```python
from build123d import *

# Parameters (mm, degrees)
PAD_DEPTH       = 8
SKETCH001_R     = 6.75
PAD001_DEPTH    = 7
SKETCH002_R     = 5.05
POCKET_DEPTH    = 15.001
SKETCH003_R     = 3.5
PAD002_DEPTH    = 5
PAD003_DEPTH    = 10
SKETCH005_W     = 15.5
SKETCH005_H     = 8
PAD004_DEPTH    = 9
SKETCH006_R     = 2.5
POCKET001_DEPTH = 31.001
POCKET002_DEPTH = 3.1


with BuildPart() as part:
    # Sketch → Pad (new body)
    with BuildSketch(Plane.XZ):
        with BuildLine():
            ThreePointArc((-28, 11), (-39, 0), (-28, -11))
            Line((-28, -11), (28, -11))
            ThreePointArc((28, -11), (39, 0), (28, 11))
            Line((-28, 11), (28, 11))
        make_face()
    extrude(amount=PAD_DEPTH)

    # Sketch001 (on Face5 of Pad) → Pad001 (join)
    with BuildSketch(Plane(origin=(0, 0, 0), x_dir=(1, 0, 0), z_dir=(0, 1, 0))):
        with Locations((-28, 0)):
            Circle(SKETCH001_R)
        with Locations((28, 0)):
            Circle(SKETCH001_R)
    extrude(amount=PAD001_DEPTH)

    # Sketch002 (on Face5 of Pad001) → Pocket (cut, through all)
    with BuildSketch(Plane.XZ.offset(8)):
        with Locations((-28, 0)):
            Circle(SKETCH002_R)
        with Locations((28, 0)):
            Circle(SKETCH002_R)
    extrude(amount=-POCKET_DEPTH, mode=Mode.SUBTRACT)

    # Sketch003 (on DatumPlane) → Pad002 (join)
    with BuildSketch(Plane.XY.offset(3.75)):
        with BuildLine():
            Line((-17.5, -8), (-6.180484, -29.286582))
            ThreePointArc((-6.180484, -29.286582), (0, -33), (6.180484, -29.286582))
            Line((17.5, -8), (6.180484, -29.286582))
            Line((-17.5, -8), (17.5, -8))
        make_face()
        with Locations((0, -26)):
            Circle(SKETCH003_R, mode=Mode.SUBTRACT)
    pad002 = extrude(amount=PAD002_DEPTH)

    # Mirrored: Pad002 across XY
    add(pad002.mirror(Plane.XY))

    # Sketch004 → Pad003 (join, symmetric)
    with BuildSketch(Plane.YZ):
        Polygon((0, 8), (0, -8), (20, 3), (20, 8), align=None)
    extrude(amount=PAD003_DEPTH, both=True)

    # Sketch005 (on Face2 of Pad003) → Pad004 (join)
    with BuildSketch(Plane(origin=(0, 0, 11), x_dir=(-1, 0, 0), z_dir=(0, 0, 1))):
        with Locations((0, 4)):
            Rectangle(SKETCH005_W, SKETCH005_H)
    extrude(amount=PAD004_DEPTH)

    # Sketch006 (on Face3 of Pad004) → Pocket001 (cut, through all)
    with BuildSketch(Plane(origin=(0, 0, -11), x_dir=(1, 0, 0), z_dir=(0, 0, -1))):
        with Locations((-4, 4)):
            Circle(SKETCH006_R)
        with Locations((4, 4)):
            Circle(SKETCH006_R)
    extrude(amount=-POCKET001_DEPTH, mode=Mode.SUBTRACT)

    # Sketch007 (on Face3 of Pocket001) → Pocket002 (cut)
    with BuildSketch(Plane(origin=(0, 0, -11), x_dir=(1, 0, 0), z_dir=(0, 0, -1))):
        Polygon((-0.55, 5.991858), (-4, 7.983717), (-7.45, 5.991858), (-7.45, 2.008142), (-4, 0.016283), (-0.55, 2.008142), align=None)
        Polygon((4, 7.983717), (0.55, 5.991858), (0.55, 2.008142), (4, 0.016283), (7.45, 2.008142), (7.45, 5.991858), align=None)
    extrude(amount=-POCKET002_DEPTH, mode=Mode.SUBTRACT)


solid = part.part
```
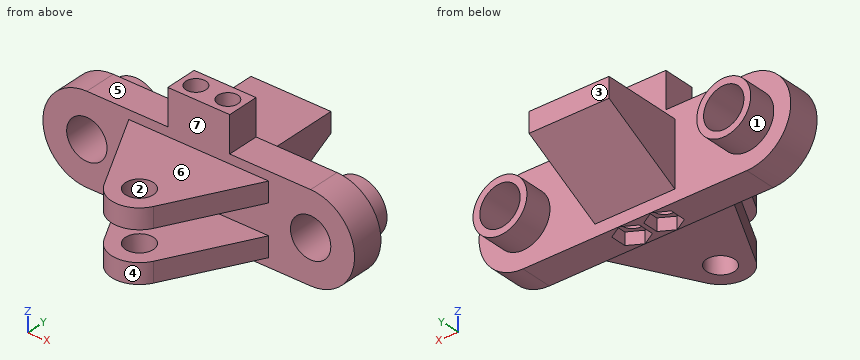
Could you check a few things on this model? Use its own coordinates, in mm. Face numbers are marked on the shaded views. A direction names the side the tool comes from. Round coordinates to 2 decimals unless told otherwise and drop trailing zeros. Loops run counter-clockwise (first coordinate to the right, second up) from the corner with the lowest first, then second, coordinate; pieces in that order, holes last.
Q1. Thinking about a two-plate mould opening in Y: for the marked faces 1, 2, 3 and 4, which applies, pulls with the +Y half, pulls with the -Y half, needs draft (parallel to the pull), parting line crosses it, or undercut?
Q2. Please list where these lines run through material, in increasing order: L1, parallel to Z at x = -4, y = -25.5; L2, parallel to Y at x = 0, z = 5.75; L3, parallel to Z at x = 28, y = 2.5.
Q3. On a 3-axis mill with a long thin cutter (end or side, diameter ignored), from which of +Z, -Z, +X, -X, +Y, -Y can I reach the whole of each face in a straight line? I mean the marked faces 5, 6 and 7. Say none if no direction works.
Q4. For P1, Ø6, axis at y = 13, z = 3, coming from the +X side; P2, Ø6, axis at y = 9, z = 0, coming from the +X side; P3, Ø0.9, axis at y = -4, z = -9.5, coming from the +X side; P4, Ø10, axis at x = 1.5, z = -3.5, coming from the -Y side, each with a flat end and sliding along its axis, tell me the tip position at first contact or that it passes through.
Q5. I want a section at D-D (y = -17). Write out the boundary of the cut face in (x, z), and give its area (3 significant figures).
Q6. I want a section at B-B (x = -24). Write out the boundary of the cut face in (y, z), and give its area (3 significant figures).
Q7. I want a section at C-C (z = 16). Write out the boundary of the cut face in (x, y), and give its area (3 significant figures).
Q8. I want a section at A-A (y = -4). Write out the boundary of the cut face in (x, z), and give its area (3 significant figures).
Answer below:
1. face 1: needs draft
1. face 2: undercut
1. face 3: pulls with the +Y half
1. face 4: pulls with the -Y half
2. L1: z = -8.75 to -3.75, 3.75 to 8.75
2. L2: y = -33 to -29.5, -22.5 to 20
2. L3: z = -6.75 to -5.05, 5.05 to 6.75
3. face 5: +Z, -X, +Y, -Y
3. face 6: +Z, +X, -X, -Y
3. face 7: -Y
4. P1: stops at x = 10
4. P2: stops at x = 34.75
4. P3: stops at x = 34.25
4. P4: stops at y = -33
5. outline: (-12.71, -8.75) - (12.71, -8.75) - (12.71, -3.75) - (-12.71, -3.75) - close; (-12.71, 3.75) - (12.71, 3.75) - (12.71, 8.75) - (-12.71, 8.75) - close
5. area: 254 mm2
6. outline: (-8, -11) - (0, -11) - (0, -5.44) - (7, -5.44) - (7, -3.08) - (-8, -3.08) - close; (-8, 3.08) - (7, 3.08) - (7, 5.44) - (0, 5.44) - (0, 11) - (-8, 11) - close
6. area: 160 mm2
7. outline: (-7.75, -8) - (7.75, -8) - (7.75, 0) - (-7.75, 0) - close; hole circle Ø5 at (-4, -4); hole circle Ø5 at (4, -4)
7. area: 84.7 mm2
8. outline: (-28, -11) - (-7.45, -11) - (-7.45, -7.9) - (-6.5, -7.9) - (-6.5, 20) - (-7.75, 20) - (-7.75, 11) - (-28, 11) arc R11 ccw to start; (-1.5, -7.9) - (-0.55, -7.9) - (-0.55, -11) - (0.55, -11) - (0.55, -7.9) - (1.5, -7.9) - (1.5, 20) - (-1.5, 20) - close; (6.5, -7.9) - (7.45, -7.9) - (7.45, -11) - (28, -11) arc R11 ccw to (28, 11) - (7.75, 11) - (7.75, 20) - (6.5, 20) - close; hole circle Ø10.1 at (-28, 0); hole circle Ø10.1 at (28, 0)
8. area: 1,270 mm2
